Here's how the part is built. I have some questions about the finished solid (model axes, mm). Coordinates: 2 decimals unless noted, no trailing zeros. Write each loop counter-clockwise with the first axis right and the second up, starting at its lowest first coordinate (ties: lowest second). Pieces come first, ordered by that corner, then holes. Notation, with made-up numbers: (-2.5, 59.5) -> (52.5, 59.5) arc R32 cw to (52.5, 85.5) -> close; hole circle Ø10 at (70.25, -21). An arc over 180 degrees is marked (long way). Put each result on its own line as item: value. Start each with the question number.
Item 1: I want a section at A-A, the plane x = 0.75. List the corners of the cut face in (y, z) for me, then the cut area to 3 significant figures.
Item 2: I need wall thicknesses on line 1 (Z direction, x = -1.25, y = 0); line 2 (X direction, y = 0.1, z = -3.2); line 3 (Y direction, x = -5, z = -0.3). Which ranges of each line are inside material? Lowest first, please. Write a range as [from, to].
Item 3: I want a section at B-B, the plane z = -1.1. State how many separate pieces and enclosed holes the cut face has, then the cut area to 3 significant figures.
Item 4: I want a section at C-C, the plane x = 3.25. List the corners of the cut face in (y, z) for me (3 decimals), then the cut area to 3 significant figures.
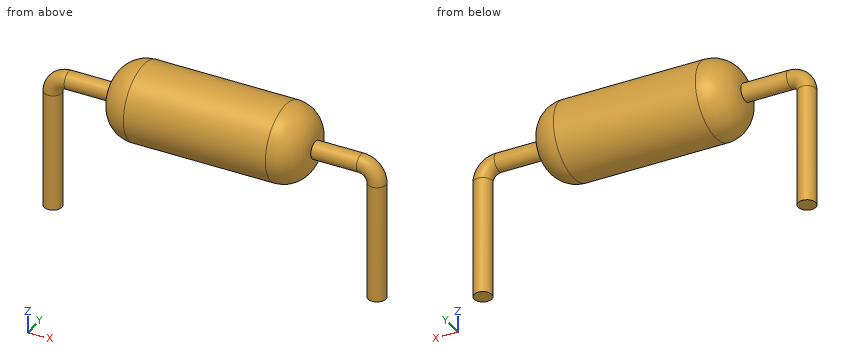
from build123d import *

# Parameters (mm, degrees)
F0_R     = 1.2
F1_DEPTH = 3.15
F2_R     = 0.925
F3_R     = 0.275


with BuildPart() as f1:
    # F0 (on Right) → F1 (new body)
    with BuildSketch(Plane.YZ):
        Circle(F0_R)
    extrude(amount=F1_DEPTH)

    # F2
    f2_edges = [f1.edges().sort_by_distance(p)[0] for p in [
        (3.15, -1.2, 0),
    ]]
    fillet(f2_edges, radius=F2_R)

    # F5: sweep along a path in F4
    with BuildLine(Plane.XZ) as f5_path:
        Line((3.15, 0), (4.58, 0))
        ThreePointArc((4.58, 0), (4.933553, -0.146447), (5.08, -0.5))
        Line((5.08, -0.5), (5.08, -4.2))
    # F3 (on face) → F5 (sweep)
    with BuildSketch(Plane.YZ.offset(3.15)):
        Circle(F3_R)
    sweep(path=f5_path.line)

    # F6: F1 across face


with BuildPart() as f1_1:
    add(f1.part)
    add(f1.part.mirror(Plane(origin=(0, 0, 0), x_dir=(0, 1, 0), z_dir=(-1, 0, 0))))


solid = f1_1.part
Calculated:
1. outline: circle Ø2.4 at (0, 0)
1. area: 4.52 mm2
2. line 1: z = [-1.2, 1.2]
2. line 2: x = [-5.34, -4.82], [4.82, 5.34]
2. line 3: y = [-0.27, 0.27]
3. separate pieces: 3
3. enclosed holes: 0
3. area: 5.37 mm2
4. outline: circle Ø0.55 at (0, 0)
4. area: 0.238 mm2
